from build123d import *

# Parameters (mm, degrees)
F1_DEPTH = 5
F2_SIZE  = 2
F3_R     = 1.2


with BuildPart() as f1:
    # F0 (on Top) → F1 (new body)
    with BuildSketch(Plane.XY):
        with BuildLine():
            Line((-120, 1.5907304411), (-103, 1.5907304411))
            Line((-103, 1.5907304411), (-103, 5.5907304411))
            Line((-103, 5.5907304411), (-112, 5.5907304411))
            Line((-112, 5.5907304411), (-112, 6.9907304411))
            Line((-112, 6.9907304411), (-62.8, 6.9907304411))
            Line((-62.8, 6.9907304411), (-62.8, 1.5907304411))
            Line((-62.8, 1.5907304411), (-59.8, 1.5907304411))
            Line((-59.8, 1.5907304411), (-56.6823085464, 6.9907304411))
            Line((-56.6823085464, 6.9907304411), (-4, 6.9907304411))
            ThreePointArc((-4, 6.9907304411), (-2.8284271247, 9.8191575658), (0, 10.9907304411))
            Line((0, 10.9907304411), (-120, 10.9907304411))
            Line((-120, 10.9907304411), (-120, 1.5907304411))
        make_face()
        with BuildLine():
            ThreePointArc((4, 6.9907304411), (2.8284271247, 9.8191575658), (0, 10.9907304411))
            Line((0, 10.9907304411), (0, 8.4907304411))
            ThreePointArc((0, 8.4907304411), (1.0606601718, 8.0513906128), (1.5, 6.9907304411))
            ThreePointArc((1.5, 6.9907304411), (0, 5.4907304411), (-1.5, 6.9907304411))
            Line((-1.5, 6.9907304411), (-4, 6.9907304411))
            ThreePointArc((-4, 6.9907304411), (0, 2.9907304411), (4, 6.9907304411))
        make_face()
        with BuildLine():
            Line((0, 8.4907304411), (0, 10.9907304411))
            ThreePointArc((0, 10.9907304411), (-2.8284271247, 9.8191575658), (-4, 6.9907304411))
            Line((-4, 6.9907304411), (-1.5, 6.9907304411))
            ThreePointArc((-1.5, 6.9907304411), (-1.0606601718, 8.0513906128), (0, 8.4907304411))
        make_face()
    extrude(amount=F1_DEPTH)

    # F2
    f2_edges = [f1.edges().sort_by_distance(p)[0] for p in [
        (0, 5.49073, 5),
        (0, 5.49073, 0),
    ]]
    chamfer(f2_edges, length=F2_SIZE)

    # F3
    f3_edges = [f1.edges().sort_by_distance(p)[0] for p in [
        (0, 8.49073, 2.5),
        (0, 5.49073, 2),
        (0, 5.49073, 3),
    ]]
    fillet(f3_edges, radius=F3_R)


solid = f1.part
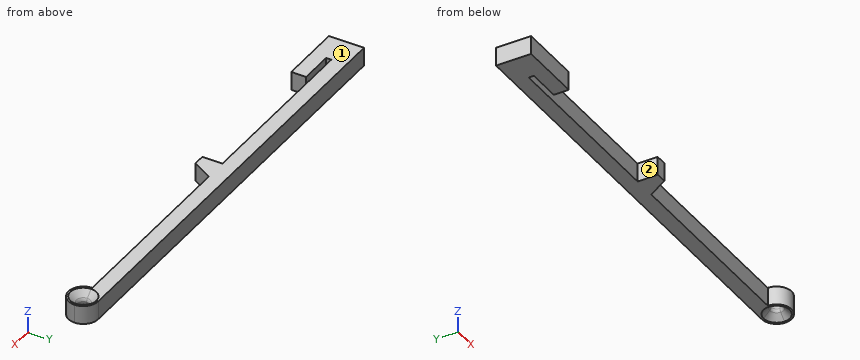
Geometry: final body of the model. Coordinates: model frame, mm. Face numbers are marked on the shaded views. A direction names the side the tool comes from. Round coordinates to 2 decimals unless told otherwise and drop trailing zeros.
Q1. Pin query (flat end, axial travel): P1, Ø1, axis at x = -77.5, z = 4, coming from the -Y side; P2, Ø0.7, axis at y = 6, z = 2.5, coming from the +X side; P3, Ø1.5, axis at y = 9.5, z = 2.5, coming from the +X side. Return the tip coordinate at first contact, or that it passes through.
Q2. Access query for the marked faces 1 and 2. Directions: +Z, -Z, +X, -X, +Y, -Y. A direction counts if a zero-diameter tool reaches every point of the face in a straight line with its end or side. Return the directions, or none.
Q3. Material intervals for L1, parallel to X at y = 4.75, z = 2.8; L2, parallel to X at y = 6.5, z = 4.3; L3, parallel to X at y = 5.5, z = 4.7, sorted ascending.
Evaluation:
1. P1: stops at y = 6.99
1. P2: stops at x = 3.95
1. P3: stops at x = 3.59
2. face 1: +Z, +X, -X, +Y, -Y
2. face 2: +Z, -Z, -Y
3. L1: x = -120 to -103, -62.8 to -57.98, -3.31 to 3.31
3. L2: x = -120 to -112, -62.8 to -56.97, -3.97 to -2.76, 2.76 to 3.97
3. L3: x = -120 to -103, -62.8 to -57.54, -3.71 to -2.83, 2.83 to 3.71
